```python
from build123d import *

# Parameters (mm, degrees)
F0_W           = 50
F0_H           = 136
F1_DEPTH       = 12
F3_D           = 15
F5_D           = 8.8
F5_CSINK_D     = 17.92
F5_CSINK_ANGLE = 90
F7_D           = 5
F7_DEPTH       = 20
F7_TIP         = 1.5021515476


with BuildPart() as f1:
    # F0 (on Top) → F1 (new body)
    with BuildSketch(Plane.XY):
        Rectangle(F0_W, F0_H)
    extrude(amount=-F1_DEPTH)

    # F3 (through all)
    with Locations(Plane.XY):
        with Locations((0, -38)):
            Hole(F3_D / 2)

    # F5 (through all)
    with Locations(Plane.XY):
        with Locations((12.5, 48), (-12.5, 48)):
            CounterSinkHole(F5_D / 2, F5_CSINK_D / 2, counter_sink_angle=F5_CSINK_ANGLE)

    # F7
    with Locations(Plane.YZ.offset(25)):
        with Locations((-38, -6)):
            Hole(F7_D / 2, depth=F7_DEPTH)
            with Locations((0, 0, -(F7_DEPTH + F7_TIP / 2))):  # 118° drill point
                Cone(0, F7_D / 2, F7_TIP, mode=Mode.SUBTRACT)


solid = f1.part
```
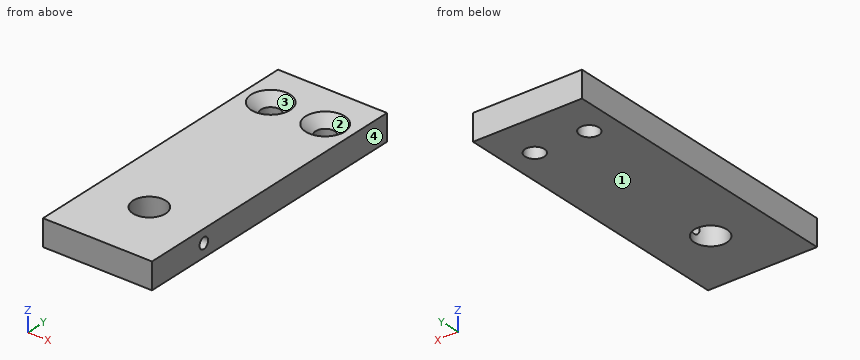
CAD build for the part. Positions are in the model's coordinates, mm. Face numbers are marked on the shaded views. Round coordinates to 2 decimals unless told otherwise and drop trailing zeros. Write each loop counter-clockwise with the first axis right and the second up, starting at its lowest first coordinate (ties: lowest second). Pieces come first, ordered by that corner, then holes.
Item 1: Mould opens along X. For the marked faces 1, 2, 3 and 4 say: released by +X, released by -X, zero draft, split by the parting line, or undercut.
Filled in:
face 1: zero draft
face 2: undercut
face 3: undercut
face 4: released by +X
Item 2: Band-saw the part on D-D on y = 48. Write the cut outline in (x, z), then the cut area to 3 significant figures.
Filled in:
outline: (-25, -12) - (-16.9, -12) - (-16.9, -4.56) - (-21.46, 0) - (-25, 0) - close; (-8.1, -12) - (8.1, -12) - (8.1, -4.56) - (3.54, 0) - (-3.54, 0) - (-8.1, -4.56) - close; (16.9, -12) - (25, -12) - (25, 0) - (21.46, 0) - (16.9, -4.56) - close
area: 347 mm2
Item 3: Band-saw the part on C-C on x = 0. Write the cut outline in (y, z).
Filled in:
outline: (-68, -12) - (-45.5, -12) - (-45.5, 0) - (-68, 0) - close; (-30.5, -12) - (68, -12) - (68, 0) - (-30.5, 0) - close
Item 4: Drill centre lines: L1, parallel to Y at x = 12.5, z = -9.25; L2, parallel to Y at x = 0, z = -5; L3, parallel to Y at x = 12.5, z = -7.5. Where is each one in solid material? Low to high.
Filled in:
L1: y = -68 to 43.6, 52.4 to 68
L2: y = -68 to -45.5, -30.5 to 68
L3: y = -68 to -40, -36 to 43.6, 52.4 to 68
Item 5: Band-saw the part on A-A on z = -9.75. Write the cut outline in (x, y), then the cut area to 3 significant figures.
Filled in:
outline: (-25, -68) - (25, -68) - (25, 68) - (-25, 68) - close; hole circle Ø8.8 at (-12.5, 48); hole circle Ø15 at (0, -38); hole circle Ø8.8 at (12.5, 48)
area: 6,500 mm2
Item 6: Band-saw the part on B-B on y = -38. Write the cut outline in (x, z), then the cut area to 4 significant figures.
Filled in:
outline: (-25, -12) - (-7.5, -12) - (-7.5, 0) - (-25, 0) - close; (7.5, -12) - (25, -12) - (25, -8.5) - (7.5, -8.5) - close; (7.5, -3.5) - (25, -3.5) - (25, 0) - (7.5, 0) - close
area: 332.5 mm2
Item 7: Drop a flat-ended pin along its axis: pin 1 Ø3 at (x, y) = (-7, 46.5) entering from +Z. Give the stop position or say it passes through.
Filled in:
pin 1: stops at z = -1.76
